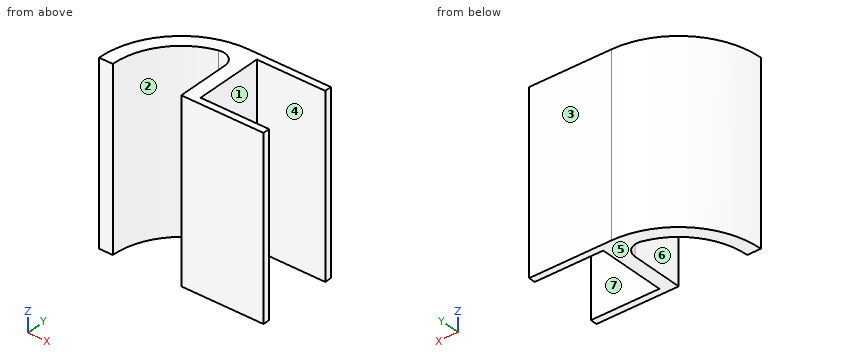
```python
from build123d import *

# Parameters (mm, degrees)
CYLINDER001_W     = 10
CYLINDER001_H     = 26
CYLINDER001_ANGLE = 90
BOX001_W          = 10
BOX001_H          = 10
BOX001_DEPTH      = 26
CYLINDER_W        = 12
CYLINDER_H        = 26
CYLINDER_ANGLE    = 90
BOX_W             = 12
BOX_H             = 12
BOX_DEPTH         = 26
FILLET_R          = 2


with BuildPart() as cylinder001:
    # Cylinder001 → Cylinder001 (revolve)
    with BuildSketch(Plane.YZ):
        with Locations((5, 13)):
            Rectangle(CYLINDER001_W, CYLINDER001_H)
    revolve(axis=Axis((0, 0, 0), (0, 0, 1)), revolution_arc=CYLINDER001_ANGLE)


with BuildPart() as cube001:
    # Box001 → Box001 (new body)
    with BuildSketch(Plane(origin=(2, 1, 0), x_dir=(1, 0, 0), z_dir=(0, 0, 1))):
        with Locations((5, 5)):
            Rectangle(BOX001_W, BOX001_H)
    extrude(amount=BOX001_DEPTH)


with BuildPart() as cylinder:
    # Cylinder → Cylinder (revolve)
    with BuildSketch(Plane.YZ):
        with Locations((6, 13)):
            Rectangle(CYLINDER_W, CYLINDER_H)
    revolve(axis=Axis((0, 0, 0), (0, 0, 1)), revolution_arc=CYLINDER_ANGLE)


with BuildPart() as fillet_body:
    # Box → Box (new body)
    with BuildSketch(Plane.XY):
        with Locations((6, 6)):
            Rectangle(BOX_W, BOX_H)
    extrude(amount=BOX_DEPTH)

    # Fusion: union Cylinder
    add(cylinder.part)

    # Cut: cut Cube001
    add(cube001.part, mode=Mode.SUBTRACT)

    # Cut001: cut Cylinder001
    add(cylinder001.part, mode=Mode.SUBTRACT)

    # Fillet
    fillet_edges = [fillet_body.edges().sort_by_distance(p)[0] for p in [
        (0, 10, 13),
    ]]
    fillet(fillet_edges, radius=FILLET_R)


solid = fillet_body.part
```
Design review of the part built by this model. Coordinates are the model's own, in mm. Face numbers are marked on the shaded views. A direction names the side the tool comes from. Coordinates: 2 decimals unless noted, no trailing zeros. Loops run counter-clockwise (first coordinate to the right, second up) from the corner with the lowest first, then second, coordinate; pieces in that order, holes last. Notation, with made-up numbers: (-23.5, 81.25) -> (19.5, 81.25) arc R14 ccw to (19.5, 99.25) -> close; hole circle Ø2 at (-28.5, 42.25). An arc over 180 degrees is marked (long way). Answer as a JSON object with one key per item and string values.
Q1. Take a section at A-A on x = 10. Give the boundary of the cut face in (y, z).
Answer block:
{"outline": "(0, 0) -> (1, 0) -> (1, 26) -> (0, 26) -> close; (11, 0) -> (12, 0) -> (12, 26) -> (11, 26) -> close"}
Q2. Take a section at C-C on y = 6.75. Give the boundary of the cut face in (x, z).
Answer block:
{"outline": "(-9.92, 0) -> (-7.38, 0) -> (-7.38, 26) -> (-9.92, 26) -> close; (0, 0) -> (2, 0) -> (2, 26) -> (0, 26) -> close"}
Q3. The part is to be moulded in two halves that separate along Y. For the marked faces 1, 2, 3 and 4, say which applies: +Y half, -Y half, draft (parallel to the pull), parting line (faces both ways), or undercut.
Answer block:
{"face 1": "undercut", "face 2": "-Y half", "face 3": "+Y half", "face 4": "undercut"}
Q4. Clearance check with flat-ended pins moving along their axes: pin 1 Ø4 at (y, z) = (4, 7.5) entering from -X; pin 2 Ø2 at (x, y) = (-9, 10.5) entering from +Z; pin 3 Ø5 at (y, z) = (7, 18.5) entering from +X; pin 4 Ø6 at (y, z) = (4, 14.5) entering from -X. State where each tip first meets the part, or that it passes through.
Answer block:
{"pin 1": "stops at x = -11.83", "pin 2": "passes through", "pin 3": "stops at x = 2", "pin 4": "stops at x = -11.96"}
Q5. To check wall thickness, follow L1, parallel to Y at x = 6.25, z = 21; L2, parallel to X at y = 1.25, z = 24.5; L3, parallel to X at y = 7, z = 23.5. State the ranges of each line that lie inside material, in increasing order.
Answer block:
{"L1": "y = 0 to 1, 11 to 12", "L2": "x = -11.93 to -9.92, 0 to 2", "L3": "x = -9.75 to -7.14, 0 to 2"}
Q6. Take a section at B-B on z = 17.5. Give the boundary of the cut face in (x, y).
Answer block:
{"outline": "(-12, 0) -> (-10, 0) arc R10 cw to (-2.5, 9.68) arc R2 cw to (0, 7.75) -> (0, 0) -> (12, 0) -> (12, 1) -> (2, 1) -> (2, 11) -> (12, 11) -> (12, 12) -> (0, 12) arc R12 ccw to start"}
Q7. Take a section at D-D on x = -9.25. Give the boundary of the cut face in (y, z), plus the area to 4 significant figures.
Answer block:
{"outline": "(3.8, 0) -> (7.64, 0) -> (7.64, 26) -> (3.8, 26) -> close", "area": "100.0 mm^2"}
Q8. Tool access review of the marked faces 5, 6 and 7: name each direction out of +Z, -Z, +X, -X, +Y, -Y from which nothing blocks a thin tool from reaching the whole face with its end or side.
Answer block:
{"face 5": "-Z, +X, -X, +Y, -Y", "face 6": "+Z, -Z, -Y", "face 7": "+Z, -Z, +X"}
